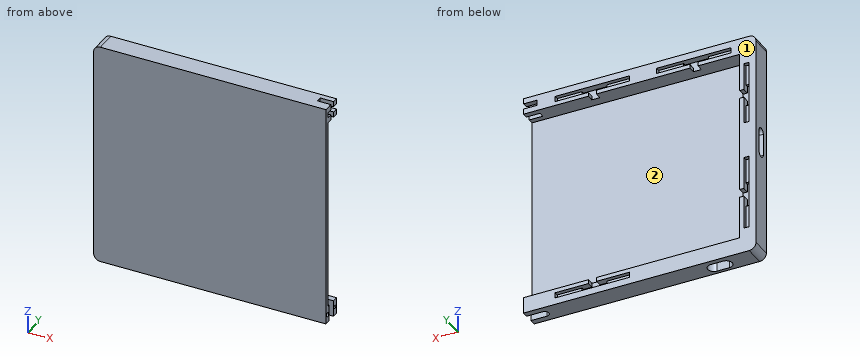
```python
from build123d import *

# Parameters (mm, degrees)
SKETCH1_W           = 159.54
SKETCH1_H           = 142.875
BOSS_EXTRUDE1_DEPTH = 3
BOSS_EXTRUDE2_DEPTH = 15
CUT_EXTRUDE1_DEPTH  = 3
CUT_EXTRUDE2_DEPTH  = 2
CUT_EXTRUDE3_DEPTH  = 12
CUT_EXTRUDE5_DEPTH  = 12
CUT_EXTRUDE6_DEPTH  = 20
CUT_EXTRUDE8_DEPTH  = 10
FILLET2_R           = 5
FILLET3_R           = 5
SKETCH11_R          = 1.5
SKETCH11_R_2        = 1.25
CUT_EXTRUDE9_DEPTH  = 10


with BuildPart() as part:
    # Sketch1 → Boss-Extrude1 (new body)
    with BuildSketch(Plane(origin=(0, 0, 0), x_dir=(1, 0, 0), z_dir=(0, 1, 0))):
        with Locations((-79.77, 0)):
            Rectangle(SKETCH1_W, SKETCH1_H)
    extrude(amount=BOSS_EXTRUDE1_DEPTH)

    # Sketch2 → Boss-Extrude2 (add)
    with BuildSketch(Plane(origin=(0, 0, 0), x_dir=(1, 0, 0), z_dir=(0, 1, 0))):
        Polygon((0, 71.4375), (0, 83.4375), (-171.54, 83.4375), (-171.54, -83.4375), (0, -83.4375), (0, -71.4375), (-159.54, -71.4375), (-159.54, 71.4375), align=None)
    extrude(amount=BOSS_EXTRUDE2_DEPTH)

    # Sketch3 → Cut-Extrude1 (cut)
    with BuildSketch(Plane(origin=(0, 15, 0), x_dir=(1, 0, 0), z_dir=(0, 1, 0))):
        Polygon((-159.54, 39.8375), (-159.54, 33.8375), (-162.54, 33.8375), (-162.54, 9.888405135), (-166.54, 9.888405135), (-166.54, 64.788405135), (-162.54, 64.788405135), (-162.54, 39.8375), align=None)
        Polygon((-23.37, -74.4375), (-47.82, -74.4375), (-47.82, -71.4375), (-53.82, -71.4375), (-53.82, -74.4375), (-78.27, -74.4375), (-78.27, -78.4375), (-23.37, -78.4375), align=None)
        Polygon((-159.54, -37.1875), (-159.54, -43.1875), (-162.54, -43.1875), (-162.54, -63.1875), (-166.54, -63.1875), (-166.54, -17.1875), (-162.54, -17.1875), (-162.54, -37.1875), align=None)
        Polygon((-98.27, -78.4375), (-98.27, -74.4375), (-122.72, -74.4375), (-122.72, -71.4375), (-128.72, -71.4375), (-128.72, -74.4375), (-153.17, -74.4375), (-153.17, -78.4375), align=None)
        Polygon((-47.82, 74.4375), (-47.82, 71.4375), (-53.82, 71.4375), (-53.82, 74.4375), (-78.27, 74.4375), (-78.27, 78.4375), (-23.37, 78.4375), (-23.37, 74.4375), align=None)
    extrude(amount=-CUT_EXTRUDE1_DEPTH, mode=Mode.SUBTRACT)

    # Sketch4 → Cut-Extrude2 (cut)
    with BuildSketch(Plane(origin=(0, 12, 0), x_dir=(1, 0, 0), z_dir=(0, 1, 0))):
        Polygon((-53.82, 74.4375), (-53.82, 71.4375), (-47.82, 71.4375), (-47.82, 74.4375), (-41.7075, 74.4375), (-41.7075, 78.4375), (-50.82, 78.4375), (-59.9325, 78.4375), (-59.9325, 74.4375), align=None)
        Polygon((-159.54, 39.8375), (-159.54, 33.8375), (-162.54, 33.8375), (-162.54, 27.850226284), (-166.54, 27.850226284), (-166.54, 46.075226284), (-162.54, 46.075226284), (-162.54, 39.8375), align=None)
        Polygon((-166.54, -32.1875), (-166.54, -48.1875), (-162.54, -48.1875), (-162.54, -43.1875), (-159.54, -43.1875), (-159.54, -37.1875), (-162.54, -37.1875), (-162.54, -32.1875), align=None)
        Polygon((-128.72, -71.4375), (-128.72, -74.4375), (-134.8325, -74.4375), (-134.8325, -78.4375), (-116.6075, -78.4375), (-116.6075, -74.4375), (-122.72, -74.4375), (-122.72, -71.4375), align=None)
        Polygon((-53.82, -74.4375), (-59.9325, -74.4375), (-59.9325, -78.4375), (-41.7075, -78.4375), (-41.7075, -74.4375), (-47.82, -74.4375), (-47.82, -71.4375), (-53.82, -71.4375), align=None)
    extrude(amount=-CUT_EXTRUDE2_DEPTH, mode=Mode.SUBTRACT)

    # Sketch5 → Cut-Extrude3 (cut)
    with BuildSketch(Plane.ZY.offset(171.54)):
        with BuildLine():
            Line((-4.6875, 10.5), (11.6925, 10.5))
            ThreePointArc((11.6925, 10.5), (14.6925, 7.5), (11.6925, 4.5))
            Line((11.6925, 4.5), (-4.6875, 4.5))
            ThreePointArc((-4.6875, 4.5), (-7.6875, 7.5), (-4.6875, 10.5))
        make_face()
    extrude(amount=-CUT_EXTRUDE3_DEPTH, mode=Mode.SUBTRACT)

    # Sketch7 → Cut-Extrude5 (cut)
    with BuildSketch(Plane(origin=(0, 0, -83.4375), x_dir=(-1, 0, 0), z_dir=(0, 0, -1))):
        with BuildLine():
            Line((-4.5375, 10.634328206), (11.8425, 10.634328206))
            ThreePointArc((11.8425, 10.634328206), (14.8425, 7.634328206), (11.8425, 4.634328206))
            Line((11.8425, 4.634328206), (-4.5375, 4.634328206))
            ThreePointArc((-4.5375, 4.634328206), (-7.5375, 7.634328206), (-4.5375, 10.634328206))
        make_face()
    extrude(amount=-CUT_EXTRUDE5_DEPTH, mode=Mode.SUBTRACT)

    # Sketch8 → Cut-Extrude6 (cut)
    with BuildSketch(Plane(origin=(0, 0, -83.4375), x_dir=(-1, 0, 0), z_dir=(0, 0, -1))):
        with BuildLine():
            Line((136.4, 11.4), (145.4, 11.4))
            ThreePointArc((145.4, 11.4), (149.9, 6.9), (145.4, 2.4))
            Line((145.4, 2.4), (136.4, 2.4))
            ThreePointArc((136.4, 2.4), (131.9, 6.9), (136.4, 11.4))
        make_face()
    extrude(amount=-CUT_EXTRUDE6_DEPTH, mode=Mode.SUBTRACT)

    # Sketch10 → Cut-Extrude8 (cut)
    with BuildSketch(Plane(origin=(0, 0, 0), x_dir=(0, 0, -1), z_dir=(1, 0, 0))):
        Polygon((-79.4375, 15), (-75.4375, 15), (-75.4375, 11), (-71.4375, 11), (-71.4375, 7), (-75.4375, 7), (-75.4375, 3), (-79.4375, 3), (-79.4375, 7), (-83.4375, 7), (-83.4375, 11), (-79.4375, 11), align=None)
    extrude(amount=-CUT_EXTRUDE8_DEPTH, mode=Mode.SUBTRACT)

    # Fillet2
    fillet2_edges = [part.edges().sort_by_distance(p)[0] for p in [
        (-171.54, 7.5, 83.4375),
    ]]
    fillet(fillet2_edges, radius=FILLET2_R)

    # Fillet3
    fillet3_edges = [part.edges().sort_by_distance(p)[0] for p in [
        (-171.54, 7.5, -83.4375),
    ]]
    fillet(fillet3_edges, radius=FILLET3_R)

    # Sketch11 → Cut-Extrude9 (cut)
    with BuildSketch(Plane(origin=(0, 0, 0), x_dir=(0, 0, -1), z_dir=(1, 0, 0))):
        with Locations((77.4375, 2.317164103)):
            Circle(SKETCH11_R)
        with Locations((77.4375, 12.817164103)):
            Circle(SKETCH11_R_2)
    extrude(amount=-CUT_EXTRUDE9_DEPTH, mode=Mode.SUBTRACT)


solid = part.part
```
The listing builds one solid part. Answer for the finished solid, in the listing's coordinates (mm). Face numbers are marked on the shaded views. Give positions to 0.01 mm unless a question says otherwise; leave off trailing zeros. Order: outer loops, then holes, each group sorted by start corner. A loop starts at its lowest first (then second) coordinate and runs counter-clockwise, first axis right, second up.
1) Find section C-C on z = -31.5. Write down the section's boundary in (x, y).
Reported:
outline: (-171.54, 0) - (0, 0) - (0, 3) - (-159.54, 3) - (-159.54, 15) - (-162.54, 15) - (-162.54, 10) - (-166.54, 10) - (-166.54, 15) - (-171.54, 15) - close
2) Consider line 1 along Z through (x, y) = (-45, 11); line 2 along Z through (x, y) = (-104.5, 14.25); line 3 along Z through (x, y) = (-68, 7). Determine where each line is inside the solid, lowest interval first.
Reported:
line 1: z = -83.44 to -78.44, -74.44 to -71.44, 71.44 to 74.44, 78.44 to 83.44
line 2: z = -83.44 to -71.44, 71.44 to 74.44, 78.44 to 83.44
line 3: z = -83.44 to -71.44, 71.44 to 83.44
3) Given P1, Ø5, axis at x = -27, z = -47.5, coming from the -Y side; P2, Ø1.8, axis at y = 2.32, z = -77.44, coming from the +X side; P3, Ø1, axis at x = -117.5, z = -10.5, coming from the +Y side; P4, Ø1.2, axis at x = -164, z = 52, coming from the +Y side, each flat-ended and moving along its own axis, determine where each tip first touches the part or whether it passes through.
Reported:
P1: stops at y = 0
P2: stops at x = -10
P3: stops at y = 3
P4: stops at y = 12
4) Find section B-B on x = -104. Write down the section's boundary in (y, z).
Reported:
outline: (0, -83.44) - (15, -83.44) - (15, -71.44) - (3, -71.44) - (3, 71.44) - (15, 71.44) - (15, 74.44) - (12, 74.44) - (12, 78.44) - (15, 78.44) - (15, 83.44) - (0, 83.44) - close
5) Find section A-A on z = 8.5. Write down the section's boundary in (x, y).
Reported:
outline: (-171.54, 0) - (0, 0) - (0, 3) - (-159.54, 3) - (-159.54, 4.5) - (-171.54, 4.5) - close; (-171.54, 10.5) - (-159.54, 10.5) - (-159.54, 15) - (-171.54, 15) - close
6) Determine the mould class of the marked faces 1 and 2 for opening direction Z: pulls with the +Z half, pulls with the -Z half, needs draft (parallel to the pull), parting line crosses it, or undercut.
Reported:
face 1: needs draft
face 2: undercut
7) Find section D-D on z = -59. Write down the section's boundary in (x, y).
Reported:
outline: (-171.54, 0) - (0, 0) - (0, 3) - (-159.54, 3) - (-159.54, 15) - (-162.54, 15) - (-162.54, 12) - (-166.54, 12) - (-166.54, 15) - (-171.54, 15) - close
